Verification items for this drawing (mm, ordinates from the low corner). A direction names the side the tool comes from. Round coordinates to 2 decimals unless told otherwise and drop trailing zeros. Loops run counter-clockwise (first coordinate to the right, second up) from the corner with the lowest first, then second, coordinate; pieces in that order, holes last. Notation, with made-up numbers: (-23.75, 50) -> (10.25, 50) arc R20 ccw to (10.25, 80) -> close; hole circle Ø4 at (27.5, 78.25). An arc over 180 degrees is marked (long way). One line per item, written item: value. Start each with the question number.
1. Cross-section at C-C on y = 12.75. Record the cut outline in (x, z).
2. Cross-section at B-B on z = 30. Record the cut outline in (x, y).
3. Cross-section at D-D on z = 20. Record the cut outline in (x, y), then the cut area to 3 significant figures.
4. Set-up check for the marked faces 1 and 2: record each of +Z, -Z, +X, -X, +Y, -Y from which the full face is reachable in a straight line by a thin tool's end or side.
5. Release check for a two-part mould opening along Z. For the marked faces 3, 4 and 5 record: +Z half, -Z half, draft (parallel to the pull), parting line (faces both ways), or undercut.
6. Cross-section at A-A on x = 30. Record the cut outline in (y, z), then the cut area to 3 significant figures.
7. Material ranges on L1, parallel to X at y = 6.25, z = 30; L2, parallel to X at y = 13.9, z = 30; L3, parallel to Y at x = 21.5, z = 11, recorded low to high.
8. Go/stop test with flat-tipped pins: pin 1 (1 mm diameter, centred on y = 11.5, z = 44, fed in from +X); pin 2 (2 mm diameter, centred on x = 47.5, y = 4.5, fed in from +Z); pin 3 (25 mm diameter, centred on x = 30, z = 36, fed in from -Y). Record where each tip stops, or that it passes through.
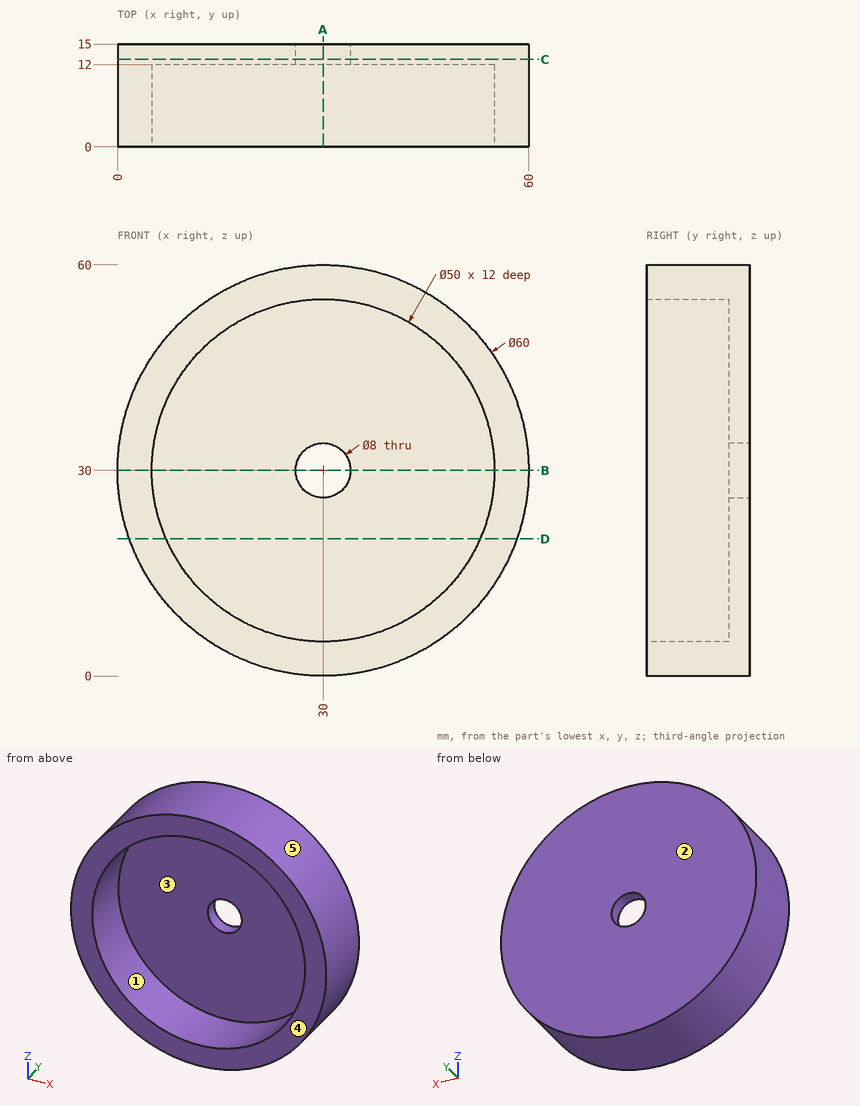
Taken from the geometry:
1. outline: circle Ø60 at (30, 30); hole circle Ø8 at (30, 30)
2. outline: (0, 0) -> (5, 0) -> (5, 12) -> (26, 12) -> (26, 15) -> (0, 15) -> close; (34, 12) -> (55, 12) -> (55, 0) -> (60, 0) -> (60, 15) -> (34, 15) -> close
3. outline: (1.72, 0) -> (7.09, 0) -> (7.09, 12) -> (52.91, 12) -> (52.91, 0) -> (58.28, 0) -> (58.28, 15) -> (1.72, 15) -> close
3. area: 299 mm2
4. face 1: -Y
4. face 2: +Z, -Z, +X, -X, +Y
5. face 3: undercut
5. face 4: draft
5. face 5: parting line
6. outline: (0, 0) -> (15, 0) -> (15, 26) -> (12, 26) -> (12, 5) -> (0, 5) -> close; (0, 55) -> (12, 55) -> (12, 34) -> (15, 34) -> (15, 60) -> (0, 60) -> close
6. area: 276 mm2
7. L1: x = 0 to 5, 55 to 60
7. L2: x = 0 to 26, 34 to 60
7. L3: y = 12 to 15
8. pin 1: stops at x = 56.79
8. pin 2: stops at z = 55.05
8. pin 3: stops at y = 12
